Here's the drawing with two shaded views (mm, measured from the low corner). I have some questions. A direction names the side the tool comes from. Coordinates: 2 decimals unless noted, no trailing zeros. Write each loop counter-clockwise with the first axis right and the second up, starting at its lowest first coordinate (ties: lowest second). Pieces come first, ordered by that corner, then holes. Notation, with made-up numbers: (14, -11.75) -> (42, -11.75) arc R19 cw to (42, 0.25) -> close; hole circle Ø10 at (-27, 5.5). An arc over 180 degrees is marked (long way). Put each result on its own line as item: value. Start each with the question number.
Item 1: I need wall thicknesses on line 1 (Z direction, x = 17, y = 5.5); line 2 (Y direction, x = 13, z = 12.75); line 3 (X direction, y = 11.5, z = 21.5). Which ranges of each line are inside material? Lowest first, please. Write a range as [from, to].
Item 2: I want a section at B-B, the plane y = 6.5. List the corners of the cut face in (x, z) for me (1 decimal).
Item 3: I want a section at A-A, the plane x = 8.75. List the corners of the cut face in (y, z) for me, then the cut area to 3 significant figures.
Item 4: If we mould it in two halves opening along Y, with no side actions, what happens to the marked faces 5, 6 and 7? For each: released by +Y, released by -Y, zero draft, split by the parting line, or undercut.
Item 5: I want a section at C-C, the plane z = 11. List the corners of the cut face in (x, y) for me.
Item 6: For pin 1 (6 mm diameter, centred on y = 2, z = 9.5, fed in from -X); pin 2 (7 mm diameter, centred on x = 10.5, z = 5, fed in from -Y); pin 3 (7 mm diameter, centred on y = 8, z = 10.5, fed in from -X); pin 4 (5 mm diameter, centred on y = 4.5, z = 4.5, fed in from +X) (1 decimal), each with a flat end and sliding along its axis, tell me the tip position at first contact or that it passes through.
Item 7: On a 3-axis mill with a long thin cutter (end or side, diameter ignored), from which of +Z, -Z, +X, -X, +Y, -Y can I reach the whole of each face in a straight line? I mean the marked faces 1, 2, 3 and 4. Say none if no direction works.
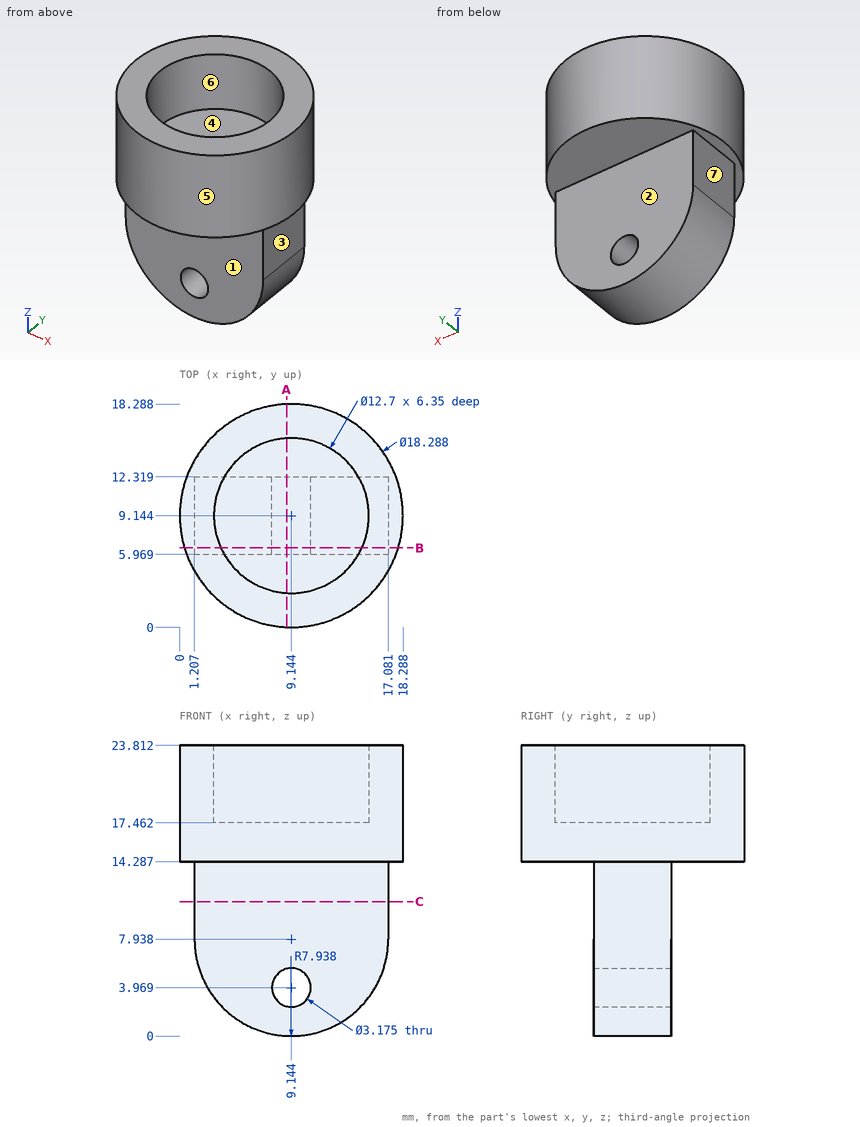
Calculated:
1. line 1: z = [14.29, 23.81]
1. line 2: y = [5.97, 12.32]
1. line 3: x = [0.31, 3.25], [15.04, 17.98]
2. outline: (0.4, 14.3) -> (1.2, 14.3) -> (1.2, 7.9) arc R7.9 ccw to (17.1, 7.9) -> (17.1, 14.3) -> (17.9, 14.3) -> (17.9, 23.8) -> (14.9, 23.8) -> (14.9, 17.5) -> (3.4, 17.5) -> (3.4, 23.8) -> (0.4, 23.8) -> close; hole circle Ø3.2 at (9.1, 4)
3. outline: (0.01, 14.29) -> (5.97, 14.29) -> (5.97, 5.51) -> (12.32, 5.51) -> (12.32, 14.29) -> (18.28, 14.29) -> (18.28, 23.81) -> (15.48, 23.81) -> (15.48, 17.46) -> (2.81, 17.46) -> (2.81, 23.81) -> (0.01, 23.81) -> close; (5.97, 0.01) -> (12.32, 0.01) -> (12.32, 2.43) -> (5.97, 2.43) -> close
3. area: 165 mm2
4. face 5: split by the parting line
4. face 6: undercut
4. face 7: zero draft
5. outline: (1.21, 5.97) -> (17.08, 5.97) -> (17.08, 12.32) -> (1.21, 12.32) -> close
6. pin 1: passes through
6. pin 2: stops at y = 5.97
6. pin 3: stops at x = 1.21
6. pin 4: stops at x = 17
7. face 1: -Z, +X, -X, -Y
7. face 2: -Z, +X, -X, +Y
7. face 3: -Z, +X, +Y, -Y
7. face 4: +Z
